Geometry: final body of the model. Coordinates: model frame, mm. Round coordinates to 2 decimals unless told otherwise and drop trailing zeros. Loops run counter-clockwise (first coordinate to the right, second up) from the corner with the lowest first, then second, coordinate; pieces in that order, holes last. Notation, with made-up numbers: M -21,5 L 11,5 A13 cw 11,30 Z; hole C 34,-13.75 d6. An arc over 180 degrees is marked long. Write each question's results on one line, items separated by ' | '.
```python
from build123d import *

# Parameters (mm, degrees)
SKETCH1_W                 = 39.5
SKETCH1_H                 = 60
BOSS_EXTRUDE1_DEPTH       = 3
SKETCH2_R                 = 2.55
CUT_EXTRUDE1_DEPTH        = 4
SKETCH4_R                 = 2.55
CUT_EXTRUDE2_DEPTH        = 4
LPATTERN1_COUNT           = 2
LPATTERN1_PITCH           = 10
LPATTERN1_COL_COUNT       = 2
LPATTERN1_COL_PITCH       = 10
LPATTERN2_COUNT           = 2
LPATTERN2_PITCH           = 20
LPATTERN2_COPY_1_SKETCH_R = 2.55
LPATTERN2_COPY_1_DEPTH    = 4
LPATTERN2_COPY_2_SKETCH_R = 2.55
LPATTERN2_COPY_2_DEPTH    = 4
FILLET1_R                 = 5
FILLET2_R                 = 5
FILLET3_R                 = 5
FILLET4_R                 = 5


with BuildPart() as part:
    # Sketch1 → Boss-Extrude1 (new body)
    with BuildSketch(Plane(origin=(0, 0, 0), x_dir=(1, 0, 0), z_dir=(0, 1, 0))):
        Rectangle(SKETCH1_W, SKETCH1_H)
    extrude(amount=BOSS_EXTRUDE1_DEPTH)

    # Sketch2 → Cut-Extrude1 (cut, through all)
    with BuildSketch(Plane(origin=(0, 3, 0), x_dir=(1, 0, 0), z_dir=(0, 1, 0))):
        with Locations((0, 21.79)):
            Circle(SKETCH2_R)
    cut_extrude1 = extrude(amount=-CUT_EXTRUDE1_DEPTH, mode=Mode.SUBTRACT)

    # Sketch4 → Cut-Extrude2 (cut, through all)
    with BuildSketch(Plane(origin=(0, 3, 0), x_dir=(1, 0, 0), z_dir=(0, 1, 0))):
        with Locations((0, -23)):
            Circle(SKETCH4_R)
    extrude(amount=-CUT_EXTRUDE2_DEPTH, mode=Mode.SUBTRACT)

    # LPattern1: Cut-Extrude1 ×2
    with Locations(*[(-i * LPATTERN1_PITCH, 0, 0) for i in range(1, LPATTERN1_COUNT)]):
        add(cut_extrude1, mode=Mode.SUBTRACT)

    # LPattern1 col: Cut-Extrude1 ×2
    with Locations(*[(i * LPATTERN1_COL_PITCH, 0, 0) for i in range(1, LPATTERN1_COL_COUNT)]):
        add(cut_extrude1, mode=Mode.SUBTRACT)

    # LPattern2: Cut-Extrude1 ×2
    with Locations(*[(0, 0, i * LPATTERN2_PITCH) for i in range(1, LPATTERN2_COUNT)]):
        add(cut_extrude1, mode=Mode.SUBTRACT)

    # LPattern2 copy 1 sketch → LPattern2 copy 1 (cut, through all)
    with BuildSketch(Plane(origin=(-10, 3, 20), x_dir=(1, 0, 0), z_dir=(0, 1, 0))):
        with Locations((0, 21.79)):
            Circle(LPATTERN2_COPY_1_SKETCH_R)
    extrude(amount=-LPATTERN2_COPY_1_DEPTH, mode=Mode.SUBTRACT)

    # LPattern2 copy 2 sketch → LPattern2 copy 2 (cut, through all)
    with BuildSketch(Plane(origin=(10, 3, 20), x_dir=(1, 0, 0), z_dir=(0, 1, 0))):
        with Locations((0, 21.79)):
            Circle(LPATTERN2_COPY_2_SKETCH_R)
    extrude(amount=-LPATTERN2_COPY_2_DEPTH, mode=Mode.SUBTRACT)

    # Fillet1
    fillet1_edges = [part.edges().sort_by_distance(p)[0] for p in [
        (-19.75, 1.5, 30),
    ]]
    fillet(fillet1_edges, radius=FILLET1_R)

    # Fillet2
    fillet2_edges = [part.edges().sort_by_distance(p)[0] for p in [
        (19.75, 1.5, -30),
    ]]
    fillet(fillet2_edges, radius=FILLET2_R)

    # Fillet3
    fillet3_edges = [part.edges().sort_by_distance(p)[0] for p in [
        (19.75, 1.5, 30),
    ]]
    fillet(fillet3_edges, radius=FILLET3_R)

    # Fillet4
    fillet4_edges = [part.edges().sort_by_distance(p)[0] for p in [
        (-19.75, 1.5, -30),
    ]]
    fillet(fillet4_edges, radius=FILLET4_R)


solid = part.part
```
1. Ray query, probe 1 along Z at (x, y) = (-10, 1); probe 2 along X at (y, z) = (0.85, -21.79); probe 3 along Z at (x, y) = (0, 1.2). Return the intervals inside material, ascending.
Answer key:
probe 1: z = -30 to -24.34, -19.24 to -4.34, 0.76 to 30 | probe 2: x = -19.75 to -12.55, -7.45 to -2.55, 2.55 to 7.45, 12.55 to 19.75 | probe 3: z = -30 to -24.34, -19.24 to -4.34, 0.76 to 20.45, 25.55 to 30
2. Draft query along Z for faces 1 (the face through (1.18, 1.52, 0.47)), 2 (the face through (18.25, 1.52, -28.57)), 3 (the face through (-5, 0, 0)), 4 (the face through (-18.32, 1.52, 28.5)). Return one class per face: pulls with the +Z half, pulls with the -Z half, needs draft (parallel to the pull), parting line crosses it, or undercut.
Answer key:
face 1: undercut | face 2: pulls with the -Z half | face 3: needs draft | face 4: pulls with the +Z half
3. Section B-B (z = -1.79). Output: boundary loops of the cut face in (x, y).
Answer key:
outline: M -19.75,0 L -12.55,0 L -12.55,3 L -19.75,3 Z; M -7.45,0 L -2.55,0 L -2.55,3 L -7.45,3 Z; M 2.55,0 L 7.45,0 L 7.45,3 L 2.55,3 Z; M 12.55,0 L 19.75,0 L 19.75,3 L 12.55,3 Z
4. Pin query (flat end, axial travel): P1, Ø6, axis at x = 10, z = -21.79, coming from the -Y side. Return the tip coordinate at first contact, or that it passes through.
Answer key:
P1: stops at y = 0
5. Section A-A (x = -10). Output: boundary loops of the cut face in (y, z), then the cut area to 3 significant figures.
Answer key:
outline: M 0,-30 L 3,-30 L 3,-24.34 L 0,-24.34 Z; M 0,-19.24 L 3,-19.24 L 3,-4.34 L 0,-4.34 Z; M 0,0.76 L 3,0.76 L 3,30 L 0,30 Z | area: 149 mm²
6. Section D-D (z = 23). Output: boundary loops of the cut face in (x, y).
Answer key:
outline: M -19.75,0 L -2.55,0 L -2.55,3 L -19.75,3 Z; M 2.55,0 L 19.75,0 L 19.75,3 L 2.55,3 Z
7. Section C-C (y = 1.7). Output: boundary loops of the cut face in (x, z), then the cut area to 3 significant figures.
Answer key:
outline: M -19.75,-25 A5 ccw -14.75,-30 L 14.75,-30 A5 ccw 19.75,-25 L 19.75,25 A5 ccw 14.75,30 L -14.75,30 A5 ccw -19.75,25 Z; hole C -10,-21.79 d5.1; hole C -10,-1.79 d5.1; hole C 0,-21.79 d5.1; hole C 0,-1.79 d5.1; hole C 0,23 d5.1; hole C 10,-21.79 d5.1; hole C 10,-1.79 d5.1 | area: 2,210 mm²
